Work out the finished part from the listing and answer in its coordinate system (mm). Face numbers are marked on the shaded views. Coordinates: 2 decimals unless noted, no trailing zeros. Write each loop counter-clockwise with the first axis right and the second up, starting at its lowest first coordinate (ties: lowest second). Pieces come first, ordered by that corner, then holes. Notation, with made-up numbers: M -20,46 L 8,46 A19 cw 8,79 Z; hole C -2,-13 d7. An arc over 180 degrees is marked long. Use CSV: the item, a comma, the result in double quotes.
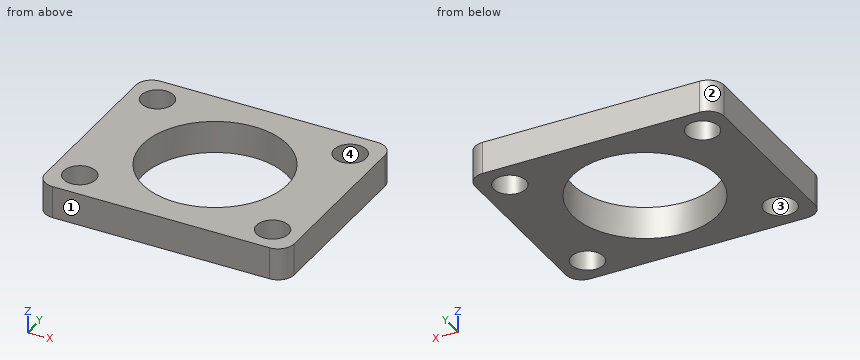
from build123d import *

# Parameters (mm, degrees)
F0_R     = 6.35
F0_R_2   = 28.575
F1_DEPTH = 12.7


with BuildPart() as f1:
    # F0 (on Top) → F1 (new body)
    with BuildSketch(Plane.XY):
        with BuildLine():
            ThreePointArc((49.2125, 33.3375), (47.352628, 37.827628), (42.8625, 39.6875))
            Line((42.8625, 39.6875), (-42.8625, 39.6875))
            ThreePointArc((-42.8625, 39.6875), (-47.352628, 37.827628), (-49.2125, 33.3375))
            Line((-49.2125, 33.3375), (-49.2125, -33.3375))
            ThreePointArc((-49.2125, -33.3375), (-47.352628, -37.827628), (-42.8625, -39.6875))
            Line((-42.8625, -39.6875), (42.8625, -39.6875))
            ThreePointArc((42.8625, -39.6875), (47.352628, -37.827628), (49.2125, -33.3375))
            Line((49.2125, -33.3375), (49.2125, 33.3375))
        make_face()
        with Locations((-38.0873, -28.5623)):
            Circle(F0_R, mode=Mode.SUBTRACT)
        with Locations((38.0873, -28.5623)):
            Circle(F0_R, mode=Mode.SUBTRACT)
        with Locations((-38.0873, 28.575)):
            Circle(F0_R, mode=Mode.SUBTRACT)
        Circle(F0_R_2, mode=Mode.SUBTRACT)
        with Locations((38.0873, 28.5623)):
            Circle(F0_R, mode=Mode.SUBTRACT)
    extrude(amount=F1_DEPTH)


solid = f1.part
Item 1: For a pull along Y with two mould halves and no side action, classify the marked faces 1, 2, 3 and 4 as released by +Y, released by -Y, zero draft, split by the parting line, or undercut.
Answer:
face 1,"released by -Y"
face 2,"released by +Y"
face 3,"undercut"
face 4,"undercut"
Item 2: The part is cut by section A-A (y = 0). Write down the section's boundary in (x, z) (1 decimal), then the cut area to 3 significant figures.
Answer:
outline,"M -49.2,0 L -28.6,0 L -28.6,12.7 L -49.2,12.7 Z; M 28.6,0 L 49.2,0 L 49.2,12.7 L 28.6,12.7 Z"
area,"524 mm2"
Item 3: The part is cut by section D-D (z = 5.5). Count the separate pieces of the cut face and the enclosed holes in it, then the cut area to 3 significant figures.
Answer:
separate pieces,"1"
enclosed holes,"5"
area,"4,710 mm2"
Item 4: Consider probe 1 along Y at (x, z) = (38, 6.5); probe 2 along Y at (x, z) = (43.5, 3.75); probe 3 along X at (y, z) = (-24, 12.25). Determine where each line is inside the solid, lowest interval first.
Answer:
probe 1,"y = -39.69 to -34.91, -22.21 to 22.21, 34.91 to 39.69"
probe 2,"y = -39.66 to -31.88, -25.24 to 25.24, 31.88 to 39.66"
probe 3,"x = -49.21 to -42.5, -33.67 to -15.51, 15.51 to 33.67, 42.5 to 49.21"
Item 5: The part is cut by section C-C (x = 40). Write down the section's boundary in (y, z), then the cut area to 3 significant figures.
Answer:
outline,"M -39.69,0 L -34.62,0 L -34.62,12.7 L -39.69,12.7 Z; M -22.51,0 L 22.51,0 L 22.51,12.7 L -22.51,12.7 Z; M 34.62,0 L 39.69,0 L 39.69,12.7 L 34.62,12.7 Z"
area,"700 mm2"
Item 6: The part is cut by section B-B (x = 0). Write down the section's boundary in (y, z) (1 decimal), then the cut area to 3 significant figures.
Answer:
outline,"M -39.7,0 L -28.6,0 L -28.6,12.7 L -39.7,12.7 Z; M 28.6,0 L 39.7,0 L 39.7,12.7 L 28.6,12.7 Z"
area,"282 mm2"
Item 7: Given pin 1 (11.5 mm diameter, centred on x = 38.09, y = -28.56, fed in from -Z), flat-ended and moving along its own axis, determine where the tip first touches the part or whether it passes through.
Answer:
pin 1,"passes through"
